```python
from build123d import *

# Parameters (mm, degrees)
SKETCH1_R           = 49
SKETCH1_R_2         = 2
BOSS_EXTRUDE1_DEPTH = 6
SKETCH3_W           = 25
SKETCH3_H           = 68
BOSS_EXTRUDE2_DEPTH = 60
CUT_EXTRUDE1_DEPTH  = 14
SKETCH5_R           = 2.4
CUT_EXTRUDE2_DEPTH  = 20
CUT_EXTRUDE3_DEPTH  = 30
CUT_EXTRUDE5_DEPTH  = 10
SKETCH13_R          = 7.5
BOSS_EXTRUDE3_DEPTH = 3
FILLET2_R           = 30
FILLET3_R           = 2
FILLET4_R           = 4


with BuildPart() as part:
    # Sketch1 → Boss-Extrude1 (new body)
    with BuildSketch(Plane(origin=(0, 0, 0), x_dir=(1, 0, 0), z_dir=(0, 1, 0))):
        with Locations(Location((0, 0, 0), (0, 0, 270))):
            Circle(SKETCH1_R)
        with Locations(Location((0, 16.5, 0), (0, 0, 270))):
            Circle(SKETCH1_R_2, mode=Mode.SUBTRACT)
        with Locations(Location((0, -16.5, 0), (0, 0, 270))):
            Circle(SKETCH1_R_2, mode=Mode.SUBTRACT)
        with Locations(Location((0, 0, 0), (0, 0, 270))):
            Circle(SKETCH1_R_2, mode=Mode.SUBTRACT)
    extrude(amount=BOSS_EXTRUDE1_DEPTH)

    # Sketch3 → Boss-Extrude2 (add)
    with BuildSketch(Plane(origin=(0, 6, 0), x_dir=(1, 0, 0), z_dir=(0, 1, 0))):
        with Locations((-17.5, 0)):
            Rectangle(SKETCH3_W, SKETCH3_H)
    extrude(amount=BOSS_EXTRUDE2_DEPTH)

    # Sketch4 → Cut-Extrude1 (cut)
    with BuildSketch(Plane.ZY.offset(30)):
        Polygon((-13.82509047, 9), (-29, 22.02774427), (6.17490953, 63), (21.349819059, 49.97225573), align=None)
    extrude(amount=-CUT_EXTRUDE1_DEPTH, mode=Mode.SUBTRACT)

    # Sketch5 → Cut-Extrude2 (cut)
    with BuildSketch(Plane.ZY.offset(16)):
        with Locations((-22.960549625, 21.386659614)):
            Circle(SKETCH5_R)
        with Locations((-15.33906677, 14.912634661)):
            Circle(SKETCH5_R)
        with Locations((7.595246131, 57.167755541)):
            Circle(SKETCH5_R)
        with Locations((15.182700896, 50.653883406)):
            Circle(SKETCH5_R)
        Polygon((-24.440289505, 27.338962606), (-9.265379976, 14.311218335), (16.790108565, 44.661037394), (1.615199035, 57.688781665), align=None)
    extrude(amount=-CUT_EXTRUDE2_DEPTH, mode=Mode.SUBTRACT)

    # Sketch8 → Cut-Extrude3 (cut)
    with BuildSketch(Plane.ZY.offset(30)):
        with BuildLine():
            Line((-34, 36), (-34, 66))
            Line((-34, 66), (0, 66))
            ThreePointArc((0, 66), (-21.05469299, 55.595318722), (-34, 36))
        make_face()
        with BuildLine():
            Line((14.5, 66), (34, 66))
            Line((34, 66), (34, 46.5))
            ThreePointArc((34, 46.5), (25.780574394, 57.780574394), (14.5, 66))
        make_face()
    extrude(amount=-CUT_EXTRUDE3_DEPTH, mode=Mode.SUBTRACT)

    # Sketch12 → Cut-Extrude5 (cut)
    with BuildSketch(Plane.ZY.offset(30)):
        with BuildLine():
            Line((-31, 6), (-31, 36))
            ThreePointArc((-31, 36), (-18.763387337, 53.246852127), (0, 63))
            Line((0, 63), (14.5, 63))
            ThreePointArc((14.5, 63), (23.838103281, 55.838103281), (31, 46.5))
            Line((31, 46.5), (31, 6))
            Line((31, 6), (-31, 6))
        make_face()
    extrude(amount=-CUT_EXTRUDE5_DEPTH, mode=Mode.SUBTRACT)

    # Sketch13 → Boss-Extrude3 (add)
    with BuildSketch(Plane(origin=(-5, 0, 0), x_dir=(0, 0, -1), z_dir=(1, 0, 0))):
        Polygon((-1.615199035, 57.688781665), (-16.790108565, 44.661037394), (9.265379976, 14.311218335), (24.440289505, 27.338962606), align=None)
        with Locations((10.338962606, 28.412545235)):
            Circle(SKETCH13_R, mode=Mode.SUBTRACT)
    extrude(amount=-BOSS_EXTRUDE3_DEPTH)

    # Fillet2
    # the kernel refuses this fillet: 30 mm, written as the material it takes off along each edge
    with BuildSketch(Plane(origin=(-70.677664467, 46.5, 34), x_dir=(0, -1, 0), z_dir=(1, 0, 0))) as fillet2_piece_1:
        with BuildLine():
            CenterArc((9.394104212, 30), FILLET2_R, 222.011677285, 47.988322715)
            ThreePointArc((-12.896148883, 9.921538481), (-6.900227571, 4.373054534), (0, 0))
            Line((0, 0), (9.394104212, 0))
        make_face()
    extrude(amount=106.355328934, mode=Mode.SUBTRACT)
    with BuildSketch(Plane(origin=(-70.677664467, 66, 14.5), x_dir=(0, -0.6097657406745188, 0.7925816938963802), z_dir=(1, 0, 0))) as fillet2_piece_2:
        with BuildLine():
            CenterArc((10.847377191, 29.50565373), FILLET2_R, 232.427433582, 47.988322715)
            Line((-7.445595029, 5.728202913), (0, 0))
            ThreePointArc((0, 0), (8.135532893, -0.741519405), (16.271065787, 0))
        make_face()
    extrude(amount=106.355328934, mode=Mode.SUBTRACT)
    with BuildSketch(Plane(origin=(-46.165023977, 66, 0), x_dir=(0, 0, 1), z_dir=(1, 0, 0))) as fillet2_piece_3:
        with BuildLine():
            CenterArc((3.733152378, 30), FILLET2_R, 250.589019729, 19.410980271)
            ThreePointArc((-6.237104224, 1.705230461), (-3.149219616, 0.740444809), (0, 0))
            Line((0, 0), (3.733152378, 0))
        make_face()
    extrude(amount=57.330047955, mode=Mode.SUBTRACT)
    with BuildSketch(Plane(origin=(-56.823799316, 36, -34), x_dir=(0, -1, 0), z_dir=(1, 0, 0))) as fillet2_piece_4:
        with BuildLine():
            CenterArc((6.194691102, -30), FILLET2_R, 90, 32.01758898)
            ThreePointArc((-9.710696233, -4.563438642), (-4.991844582, -1.99126385), (0, 0))
            Line((0, 0), (6.194691102, 0))
        make_face()
    extrude(amount=78.647598632, mode=Mode.SUBTRACT)

    # Fillet3
    fillet3_edges = [part.edges().sort_by_distance(p)[0] for p in [
        (-30, 6, 32.5),
        (-20, 6, 0),
        (-25, 6, 31),
        (-25, 6, -31),
        (-30, 6, -32.5),
        (-17.5, 6, 34),
        (-5, 6, 0),
        (-17.5, 6, -34),
    ]]
    fillet(fillet3_edges, radius=FILLET3_R)

    # Fillet4
    fillet4_edges = [part.edges().sort_by_distance(p)[0] for p in [
        (-25, 36, -31),
        (-25, 63, 0),
        (-25, 63, 14.5),
        (-25, 46.5, 31),
    ]]
    fillet(fillet4_edges, radius=FILLET4_R)


solid = part.part
```
Can you work these out from the model? Positions are in its coordinate system, mm. A direction names the side the tool comes from. Give positions to 0.01 mm unless a question says otherwise; leave off trailing zeros. Write each loop counter-clockwise with the first axis right and the second up, starting at its lowest first coordinate (ties: lowest second). Pieces come first, ordered by that corner, then holes. Notation, with made-up numbers: (43, 54.5) -> (101, 54.5) arc R25 ccw to (101, 73.5) -> close; hole circle Ø4 at (-12.5, -21). An arc over 180 degrees is marked (long way). One line per item, written item: value.
Q1. Imagine slicing it at B-B on y = 26. Please give me the cut outline in (x, z), and give its area (3 significant figures).
Results found:
outline: (-30, -34) -> (-5, -34) -> (-5, -17.44) -> (-8, -17.44) -> (-8, -22.88) -> (-16, -22.88) -> (-16, -25.59) -> (-20, -25.59) -> (-20, -31) -> (-30, -31) -> close; (-30, 31) -> (-20, 31) -> (-20, 0.77) -> (-8, 0.77) -> (-8, -3.24) -> (-5, -3.24) -> (-5, 34) -> (-30, 34) -> close
area: 743 mm^2
Q2. Please list where these lines run through material, in increasing order: line 1 (Z direction, x = -26, y = 27.5); line 2 (Y direction, x = -12.5, z = 6); line 3 (Y direction, x = -43, z = 18). Write a range as [from, to].
Results found:
line 1: z = [-34, -31], [31, 34]
line 2: y = [0, 32.09], [53.92, 55.37], [58.96, 65.99]
line 3: y = [0, 6]
Q3. Imagine slicing it at D-D on z = -16.5. Give the number of separate pieces and of enclosed holes in the cut face, and give its area (3 significant figures).
Results found:
separate pieces: 4
enclosed holes: 0
area: 1,070 mm^2
Q4. We'd pull the mould along X, two halves only. Please class faces 5 (the face through (-25, 27, 31)), 6 (the face through (-30, 58.3, -12.4)), 7 (the face through (-2, 3, 0)): +X half, -X half, draft (parallel to the pull), parting line (faces both ways), or undercut.
Results found:
face 5: draft
face 6: -X half
face 7: undercut
Q5. Imagine slicing it at C-C on z = 8. Please give me the cut outline in (x, y).
Results found:
outline: (-48.34, 0) -> (48.34, 0) -> (48.34, 6) -> (-3, 6) arc R2 cw to (-5, 8) -> (-5, 54.8) -> (-16, 54.8) -> (-16, 52.21) -> (-8, 52.21) -> (-8, 34.42) -> (-20, 34.42) -> (-20, 8) arc R2 cw to (-22, 6) -> (-48.34, 6) -> close; (-30, 63) -> (-20, 63) -> (-20, 61.43) -> (-16, 61.43) -> (-16, 59.53) -> (-5, 59.53) -> (-5, 65.86) -> (-30, 65.86) -> close
Q6. Which directions (+Z, -Z, +X, -X, +Y, -Y) give clear straight access to the entire face, cutting with the end or side of a thin tool? Please do faces 1 (the face through (-12.056, 20.916, -16.959)), 2 (the face through (-10.58, 13.45, -17.24)), 3 (the face through (-5, 37, 0)), 4 (the face through (-18, 19, -34)).
Results found:
face 1: -X
face 2: +X, -X
face 3: +Z, -Z, +X, +Y
face 4: -Z, +X, -X, +Y
Q7. For P1, Ø17.5, axis at y = 48.5, z = -2, coming from the -X side; P2, Ø10, axis at y = 8.5, z = -32.5, coming from the +X side; P3, Ø3, axis at x = -25, y = 35.5, coming from the -Z side, each with a flat end and sliding along its axis, tell me the tip position at first contact or that it passes through.
Results found:
P1: stops at x = -20
P2: stops at x = 40.09
P3: stops at z = -33.71
Q8. Imagine slicing it at A-A on x = 0. Please give me the cut outline in (y, z).
Results found:
outline: (0, -49) -> (6, -49) -> (6, -18.5) -> (0, -18.5) -> close; (0, -14.5) -> (6, -14.5) -> (6, -2) -> (0, -2) -> close; (0, 2) -> (6, 2) -> (6, 14.5) -> (0, 14.5) -> close; (0, 18.5) -> (6, 18.5) -> (6, 49) -> (0, 49) -> close
